from build123d import *
from OCP.BRepFilletAPI import BRepFilletAPI_MakeChamfer

# Parameters (mm, degrees)
SKETCH1_R           = 36
SKETCH1_R_2         = 1.7
BOSS_EXTRUDE1_DEPTH = 5
SKETCH2_W           = 40
SKETCH2_H           = 75
BOSS_EXTRUDE2_DEPTH = 2.5
SKETCH3_R           = 2.75
SKETCH3_R_2         = 1.55
BOSS_EXTRUDE3_DEPTH = 4
SKETCH4_R           = 2.75
SKETCH4_R_2         = 1.55
BOSS_EXTRUDE4_DEPTH = 4
CHAMFER1_SIZE       = 1
CHAMFER1_SIZE_2     = 4
SKETCH6_W           = 20
SKETCH6_H           = 10
CUT_EXTRUDE1_DEPTH  = 91.647669578
FILLET1_R           = 3


with BuildPart() as part:
    # Sketch1 → Boss-Extrude1 (new body)
    with BuildSketch(Plane(origin=(0, 0, 0), x_dir=(1, 0, 0), z_dir=(0, 1, 0))):
        with Locations(Location((0, 0, 0), (0, 0, 270))):
            Circle(SKETCH1_R)
        with Locations(Location((0, 32, 0), (0, 0, 270))):
            Circle(SKETCH1_R_2, mode=Mode.SUBTRACT)
        with Locations(Location((27.712812921, -16, 0), (0, 0, 270))):
            Circle(SKETCH1_R_2, mode=Mode.SUBTRACT)
        with Locations(Location((-27.712812921, -16, 0), (0, 0, 270))):
            Circle(SKETCH1_R_2, mode=Mode.SUBTRACT)
    extrude(amount=BOSS_EXTRUDE1_DEPTH)

    # Sketch2 → Boss-Extrude2 (add, symmetric)
    with BuildSketch(Plane.XY):
        with Locations((0, 42.5)):
            Rectangle(SKETCH2_W, SKETCH2_H)
    extrude(amount=BOSS_EXTRUDE2_DEPTH, both=True)

    # Sketch3 → Boss-Extrude3 (add)
    # profile 1 of 4: a face of its own
    with BuildSketch(Plane.XY.offset(2.5)):
        with Locations(Location((-13.085, 75.375, 0), (0, 0, 180))):
            Circle(SKETCH3_R)
        with Locations((-13.085, 75.375)):
            Circle(SKETCH3_R_2, mode=Mode.SUBTRACT)
    # profile 2 of 4: a face of its own
    with BuildSketch(Plane.XY.offset(2.5)):
        with Locations(Location((13.085, 75.375, 0), (0, 0, 180))):
            Circle(SKETCH3_R)
        with Locations((13.085, 75.375)):
            Circle(SKETCH3_R_2, mode=Mode.SUBTRACT)
    # profile 3 of 4: a face of its own
    with BuildSketch(Plane.XY.offset(2.5)):
        with Locations(Location((13.085, 9.625, 0), (0, 0, 180))):
            Circle(SKETCH3_R)
        with Locations((13.085, 9.625)):
            Circle(SKETCH3_R_2, mode=Mode.SUBTRACT)
    # profile 4 of 4: a face of its own
    with BuildSketch(Plane.XY.offset(2.5)):
        with Locations(Location((-13.085, 9.625, 0), (0, 0, 180))):
            Circle(SKETCH3_R)
        with Locations((-13.085, 9.625)):
            Circle(SKETCH3_R_2, mode=Mode.SUBTRACT)
    extrude(amount=BOSS_EXTRUDE3_DEPTH)

    # Sketch4 → Boss-Extrude4 (add)
    # profile 1 of 4: a face of its own
    with BuildSketch(Plane(origin=(0, 0, -2.5), x_dir=(-1, 0, 0), z_dir=(0, 0, -1))):
        with Locations((-14.125, 65)):
            Circle(SKETCH4_R)
        with Locations((-14.125, 65)):
            Circle(SKETCH4_R_2, mode=Mode.SUBTRACT)
    # profile 2 of 4: a face of its own
    with BuildSketch(Plane(origin=(0, 0, -2.5), x_dir=(-1, 0, 0), z_dir=(0, 0, -1))):
        with Locations((14.125, 65)):
            Circle(SKETCH4_R)
        with Locations((14.125, 65)):
            Circle(SKETCH4_R_2, mode=Mode.SUBTRACT)
    # profile 3 of 4: a face of its own
    with BuildSketch(Plane(origin=(0, 0, -2.5), x_dir=(-1, 0, 0), z_dir=(0, 0, -1))):
        with Locations((14.125, 24.15)):
            Circle(SKETCH4_R)
        with Locations((14.125, 24.15)):
            Circle(SKETCH4_R_2, mode=Mode.SUBTRACT)
    # profile 4 of 4: a face of its own
    with BuildSketch(Plane(origin=(0, 0, -2.5), x_dir=(-1, 0, 0), z_dir=(0, 0, -1))):
        with Locations((-14.125, 24.15)):
            Circle(SKETCH4_R)
        with Locations((-14.125, 24.15)):
            Circle(SKETCH4_R_2, mode=Mode.SUBTRACT)
    extrude(amount=BOSS_EXTRUDE4_DEPTH)

    # Chamfer1
    chamfer1_edges_1 = [part.edges().sort_by_distance(p)[0] for p in [
        (-10.335, 75.375, 2.5),
    ]]
    chamfer1_side_1 = [part.faces().sort_by_distance(p)[0] for p in [
        (-10.315, 75.375, 2.5),
    ]]
    chamfer1_edges_2 = [part.edges().sort_by_distance(p)[0] for p in [
        (15.835, 75.375, 2.5),
    ]]
    chamfer1_side_2 = [part.faces().sort_by_distance(p)[0] for p in [
        (15.855, 75.375, 2.5),
    ]]
    chamfer1_edges_3 = [part.edges().sort_by_distance(p)[0] for p in [
        (15.835, 9.625, 2.5),
    ]]
    chamfer1_side_3 = [part.faces().sort_by_distance(p)[0] for p in [
        (15.855, 9.625, 2.5),
    ]]
    chamfer1_edges_4 = [part.edges().sort_by_distance(p)[0] for p in [
        (-10.335, 9.625, 2.5),
    ]]
    chamfer1_side_4 = [part.faces().sort_by_distance(p)[0] for p in [
        (-10.315, 9.625, 2.5),
    ]]
    chamfer1_edges_5 = [part.edges().sort_by_distance(p)[0] for p in [
        (-11.375, 65, -2.5),
    ]]
    chamfer1_side_5 = [part.faces().sort_by_distance(p)[0] for p in [
        (-11.355, 65, -2.5),
    ]]
    chamfer1_edges_6 = [part.edges().sort_by_distance(p)[0] for p in [
        (16.875, 65, -2.5),
    ]]
    chamfer1_side_6 = [part.faces().sort_by_distance(p)[0] for p in [
        (16.895, 65, -2.5),
    ]]
    chamfer1_edges_7 = [part.edges().sort_by_distance(p)[0] for p in [
        (-11.375, 24.15, -2.5),
    ]]
    chamfer1_side_7 = [part.faces().sort_by_distance(p)[0] for p in [
        (-11.355, 24.15, -2.5),
    ]]
    chamfer1_edges_8 = [part.edges().sort_by_distance(p)[0] for p in [
        (16.875, 24.15, -2.5),
    ]]
    chamfer1_side_8 = [part.faces().sort_by_distance(p)[0] for p in [
        (16.895, 24.15, -2.5),
    ]]
    chamfer1 = BRepFilletAPI_MakeChamfer(part.part.solid().wrapped)
    for e in chamfer1_edges_1:
        chamfer1.Add(CHAMFER1_SIZE - 0.0001, CHAMFER1_SIZE_2 - 0.0001, e.wrapped, chamfer1_side_1[0].wrapped)
    for e in chamfer1_edges_2:
        chamfer1.Add(CHAMFER1_SIZE - 0.0001, CHAMFER1_SIZE_2 - 0.0001, e.wrapped, chamfer1_side_2[0].wrapped)
    for e in chamfer1_edges_3:
        chamfer1.Add(CHAMFER1_SIZE - 0.0001, CHAMFER1_SIZE_2 - 0.0001, e.wrapped, chamfer1_side_3[0].wrapped)
    for e in chamfer1_edges_4:
        chamfer1.Add(CHAMFER1_SIZE - 0.0001, CHAMFER1_SIZE_2 - 0.0001, e.wrapped, chamfer1_side_4[0].wrapped)
    for e in chamfer1_edges_5:
        chamfer1.Add(CHAMFER1_SIZE - 0.0001, CHAMFER1_SIZE_2 - 0.0001, e.wrapped, chamfer1_side_5[0].wrapped)
    for e in chamfer1_edges_6:
        chamfer1.Add(CHAMFER1_SIZE - 0.0001, CHAMFER1_SIZE_2 - 0.0001, e.wrapped, chamfer1_side_6[0].wrapped)
    for e in chamfer1_edges_7:
        chamfer1.Add(CHAMFER1_SIZE - 0.0001, CHAMFER1_SIZE_2 - 0.0001, e.wrapped, chamfer1_side_7[0].wrapped)
    for e in chamfer1_edges_8:
        chamfer1.Add(CHAMFER1_SIZE - 0.0001, CHAMFER1_SIZE_2 - 0.0001, e.wrapped, chamfer1_side_8[0].wrapped)
    add(Compound.cast(chamfer1.Shape()), mode=Mode.REPLACE)  # a hair under: the kernel refuses the full size

    # Sketch6 → Cut-Extrude1 (cut, through all)
    with BuildSketch(Plane(origin=(0, 5, 0), x_dir=(1, 0, 0), z_dir=(0, 1, 0))):
        with Locations((0, 7.5)):
            Rectangle(SKETCH6_W, SKETCH6_H)
        with Locations((0, -7.5)):
            Rectangle(SKETCH6_W, SKETCH6_H)
    extrude(amount=-CUT_EXTRUDE1_DEPTH, mode=Mode.SUBTRACT)

    # Fillet1
    fillet1_edges = [part.edges().sort_by_distance(p)[0] for p in [
        (-10, 2.5, -12.5),
        (10, 2.5, -12.5),
        (-10, 2.5, 12.5),
        (10, 2.5, 12.5),
        (-20, 80, 0),
        (-20, 5, 0),
        (20, 5, 0),
        (20, 80, 0),
    ]]
    fillet(fillet1_edges, radius=FILLET1_R)


solid = part.part
Can you work these out from the model? Positions are in its coordinate system, mm. A direction names the side the tool comes from. Give positions to 0.01 mm unless a question says otherwise; leave off trailing zeros. Loops run counter-clockwise (first coordinate to the right, second up) from the corner with the lowest first, then second, coordinate; pieces in that order, holes last. Notation, with made-up numbers: (-30, -25) - (-4, -25) arc R33 cw to (-4, 10) - close; hole circle Ø2 at (79.5, 52.25). An arc over 180 degrees is marked (long way). Answer as a JSON object with one key per item and string values.
Q1. Imagine slicing it at A-A on z = 4.5. Give the number of separate pieces and of enclosed holes in the cut face, plus the area to 3 significant figures.
Geometry says:
{"separate pieces": "6", "enclosed holes": "4", "area": "360 mm²"}
Q2. If I drill on L1, parallel to Y at x = 14, z = 13.5; L2, parallel to Z at x = 17, y = 53.5; L3, parallel to X at y = 26, z = -4.5, over which ranges is the centre line in solid material (lowest first)?
Geometry says:
{"L1": "0 to 5", "L2": "-2.5 to 2.5", "L3": "-16.8 to -11.45, 11.45 to 16.8"}
Q3. Imagine slicing it at B-B on z = 16. Write out the boundary of the cut face in (x, y), plus the area to 3 significant figures.
Geometry says:
{"outline": "(-32.25, 0) - (-29.41, 0) - (-29.41, 5) - (-32.25, 5) - close; (-26.01, 0) - (26.01, 0) - (26.01, 5) - (-26.01, 5) - close; (29.41, 0) - (32.25, 0) - (32.25, 5) - (29.41, 5) - close", "area": "288 mm²"}
Q4. Which directions (+Z, -Z, +X, -X, +Y, -Y) give clear straight access to the entire face, cutting with the end or side of a thin tool? Please do faces 4 (the flat face through (-16, 24, -6.5)), 5 (the flat face through (10, 3, -6)), 6 (the flat face through (-10, 3, 6)), 7 (the flat face through (-15, 10, 6.5)).
Geometry says:
{"face 4": "-Z, +X, -X, +Y", "face 5": "+Y, -Y", "face 6": "-Y", "face 7": "+Z, +X, -X, +Y"}
Q5. Imagine slicing it at D-D on z = -32. Write out the boundary of the cut face in (x, y), plus the area to 3 significant figures.
Geometry says:
{"outline": "(-16.49, 0) - (-1.7, 0) - (-1.7, 5) - (-16.49, 5) - close; (1.7, 0) - (16.49, 0) - (16.49, 5) - (1.7, 5) - close", "area": "148 mm²"}
Q6. Will these pins go through, and if not, where does the flat tip stop? P1, Ø12, axis at x = -17.5, z = 5, coming from the +Y side; P2, Ø3.5, axis at x = -13.5, y = 23.5, coming from the -Z side; P3, Ø4.5, axis at x = 12.5, y = 9, coming from the +Z side; P4, Ø4, axis at y = 31, z = 0.5, coming from the -X side.
Geometry says:
{"P1": "y = 80", "P2": "z = -6.5", "P3": "z = 6.5", "P4": "x = -20"}
Q7. If we mould it in two halves opening along X, with no side actions, what happens to faces 1 (the cylindrical face through (9.14, 2.46, -11.6)), 2 (the cylindrical face through (-20.86, 5.9, 0.04)), 3 (the flat face through (12, 24, -6.5))? For each: pulls with the +X half, pulls with the -X half, needs draft (parallel to the pull), parting line crosses it, or undercut.
Geometry says:
{"face 1": "undercut", "face 2": "pulls with the -X half", "face 3": "needs draft"}
